from build123d import *

# Parameters (mm, degrees)
SKETCH1_W                                      = 19.05
SKETCH1_H                                      = 34.925
BOSS_EXTRUDE1_DEPTH                            = 4.7625
BOSS_EXTRUDE2_DEPTH                            = 9.525
BOSS_EXTRUDE3_DEPTH                            = 9.525
CBORE_FOR_8_BUTTON_HEAD_CAP_SCREW1_D           = 4.4958
CBORE_FOR_8_BUTTON_HEAD_CAP_SCREW1_CBORE_D     = 8.73252
CBORE_FOR_8_BUTTON_HEAD_CAP_SCREW1_CBORE_DEPTH = 2.2098
FILLET1_R                                      = 6.35
SKETCH6_R                                      = 3.175
SKETCH6_R_2                                    = 2.2479
CUT_EXTRUDE1_DEPTH                             = 3.175
FILLET2_R                                      = 3.175


with BuildPart() as part:
    # Sketch1 → Boss-Extrude1 (new, symmetric)
    with BuildSketch(Plane.XY):
        Rectangle(SKETCH1_W, SKETCH1_H)
    extrude(amount=BOSS_EXTRUDE1_DEPTH, both=True)



with BuildPart() as body_2:
    # Sketch2 → Boss-Extrude2 (new body)
    with BuildSketch(Plane.XY.offset(4.7625)):
        Polygon((9.525, 17.4625), (18.56425515, 51.197459483), (0.163368159, 56.127962292), (-8.875886991, 22.393002809), align=None)
    extrude(amount=-BOSS_EXTRUDE2_DEPTH)


with BuildPart() as part_1:
    add(part.part)

    add(body_2.part)  # Boss-Extrude3 merges body 2
    # Sketch3 → Boss-Extrude3 (add)
    with BuildSketch(Plane.XY.offset(4.7625)):
        with BuildLine():
            Line((-8.875886991, 22.393002809), (9.525, 17.4625))
            Line((9.525, 17.4625), (-9.525, 17.4625))
            ThreePointArc((-9.525, 17.4625), (-9.362024609, 19.949023962), (-8.875886991, 22.393002809))
        make_face()
    extrude(amount=-BOSS_EXTRUDE3_DEPTH)

    # CBORE for #8 Button Head Cap Screw1 (through all)
    with Locations(Plane.XY.offset(4.7625)):
        with Locations((0.038567729, -0.344238019), (0.081487695, 18.705761981), (4.970520592, 37.117710746)):
            CounterBoreHole(CBORE_FOR_8_BUTTON_HEAD_CAP_SCREW1_D / 2, CBORE_FOR_8_BUTTON_HEAD_CAP_SCREW1_CBORE_D / 2, CBORE_FOR_8_BUTTON_HEAD_CAP_SCREW1_CBORE_DEPTH)

    # Fillet1
    fillet1_edges = [part_1.edges().sort_by_distance(p)[0] for p in [
        (18.56425515, 51.197459483, 0),
        (0.163368159, 56.127962292, 0),
        (9.525, -17.4625, 0),
        (-9.525, -17.4625, 0),
        (9.525, 17.4625, 0),
    ]]
    fillet(fillet1_edges, radius=FILLET1_R)

    # Sketch6 → Cut-Extrude1 (cut)
    # profile 1 of 3: a face of its own
    with BuildSketch(Plane(origin=(0, 0, -4.7625), x_dir=(-1, 0, 0), z_dir=(0, 0, -1))):
        with Locations((-4.970520592, 37.117710746)):
            Circle(SKETCH6_R)
        with Locations(Location((-4.970520592, 37.117710746, 0), (0, 0, 180))):
            Circle(SKETCH6_R_2, mode=Mode.SUBTRACT)
    # profile 2 of 3: a face of its own
    with BuildSketch(Plane(origin=(0, 0, -4.7625), x_dir=(-1, 0, 0), z_dir=(0, 0, -1))):
        with Locations((-0.081487695, 18.705761981)):
            Circle(SKETCH6_R)
        with Locations(Location((-0.081487695, 18.705761981, 0), (0, 0, 180))):
            Circle(SKETCH6_R_2, mode=Mode.SUBTRACT)
    # profile 3 of 3: a face of its own
    with BuildSketch(Plane(origin=(0, 0, -4.7625), x_dir=(-1, 0, 0), z_dir=(0, 0, -1))):
        with Locations((-0.038567729, -0.344238019)):
            Circle(SKETCH6_R)
        with Locations(Location((-0.038567729, -0.344238019, 0), (0, 0, 180))):
            Circle(SKETCH6_R_2, mode=Mode.SUBTRACT)
    extrude(amount=-CUT_EXTRUDE1_DEPTH, mode=Mode.SUBTRACT)

    # Fillet2
    fillet2_edges = [part_1.edges().sort_by_distance(p)[0] for p in [
        (-9.525, 3.175, 4.7625),
        (-9.362024609, 19.949023962, 4.7625),
        (13.331062608, 31.666919031, 4.7625),
        (9.525, 2.75700332, 4.7625),
        (9.363811655, 53.662710888, 4.7625),
        (-5.178009884, 36.193668052, 4.7625),
        (0, -17.4625, 4.7625),
        (16.286386531, 49.882331423, 4.7625),
        (7.665128061, -15.602628061, 4.7625),
        (-7.665128061, -15.602628061, 4.7625),
        (1.47849622, 53.850093673, 4.7625),
        (9.57932513, 17.455347961, 4.7625),
    ]]
    fillet(fillet2_edges, radius=FILLET2_R)


solid = part_1.part
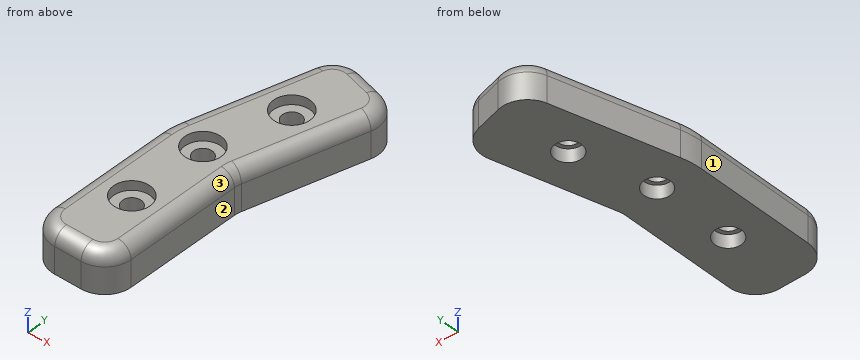
Build history of the part. All positions in model axes, mm. Face numbers are marked on the shaded views. A direction names the side the tool comes from. Give positions to 0.01 mm unless a question says otherwise; leave off trailing zeros. Answer in a Markdown table with one row per item.
Item 1: Probe line 1 along X through (y, z) = (5, 1) (3 decimals); line 2 along Y through (x, z) = (-1, -1); line 3 along X through (y, z) = (18.5, -2.75). List the from-to ranges inside material, lowest first. Write a range as [from, to].
Findings below:
| item | result |
|---|---|
| line 1 | x = [-9.525, 9.525] |
| line 2 | y = [-17.46, -2.34], [1.65, 16.74], [20.68, 51.24] |
| line 3 | x = [-9.5, -3.09], [3.25, 9.8] |
Item 2: Flat gauge pins, fed straight in: P1, Ø8, axis at x = 4.97, y = 37.12, coming from the +Z side; P2, Ø1.5, axis at y = 4, z = 2, coming from the +X side (3 decimals); P3, Ø6, axis at x = 0.08, y = 18.71, coming from the -Z side. Where does each tip first touch, or does it go through?
Findings below:
| item | result |
|---|---|
| P1 | stops at z = 2.55 |
| P2 | stops at x = 9.525 |
| P3 | stops at z = -1.59 |
Item 3: Slice it at A-A on z = -0.5. Give the number of separate pieces and of enclosed holes in the cut face, plus the area to 3 significant figures.
Findings below:
| item | result |
|---|---|
| separate pieces | 1 |
| enclosed holes | 3 |
| area | 1,300 mm² |
Item 4: Tool access for the marked faces 1, 2 and 3: list every direction of +Z, -Z, +X, -X, +Y, -Y with a clear straight run to the whole face (end or side of a thin tool).
Findings below:
| item | result |
|---|---|
| face 1 | +Z, -Z, -X, +Y, -Y |
| face 2 | +Z, -Z, +X, -Y |
| face 3 | +Z, +X, -Y |
